Check sheet for the modelled part. Datum: model origin and axes. Units: mm. A direction names the side the tool comes from. Coordinates: 2 decimals unless noted, no trailing zeros. Write each loop counter-clockwise with the first axis right and the second up, starting at its lowest first coordinate (ties: lowest second). Pieces come first, ordered by that corner, then holes. Notation, with made-up numbers: (67, 20.25) -> (105, 20.25) arc R16 ccw to (105, 39.25) -> close; hole circle Ø10 at (84, -1.75). An arc over 180 degrees is marked (long way). One line per item, written item: value. Start each with the question number.
1) Gauge pin test, flat ends, axial feed: P1, Ø5, axis at x = 6, y = -2.5, coming from the +Z side (3 decimals); P2, Ø2.5, axis at y = -2.5, z = -2.5, coming from the +X side. Record the tip position at first contact, or that the pin passes through.
2) Set-up check for faces 1 (the flat face through (12, 0, -8.255)), 2 (the flat face through (2.54, 4.762, -8.44)): record each of +Z, -Z, +X, -X, +Y, -Y from which the full face is reachable in a straight line by a thin tool's end or side.
3) Sectioned sample at B-B on y = 0. Enter the section's corners in (x, z) (1 decimal).
4) Sectioned sample at A-A on x = 15.24. Enter the section's corners in (y, z) (1 decimal), plus the area to 3 significant figures.
5) Sectioned sample at D-D on y = -4. Enter the section's corners in (x, z) (1 decimal), plus the area to 3 significant figures.
6) Draft check along Y on faces 3 (the cylindrical face through (13.09, 0.09, -10.92)), 4 (the flat face through (0, 0, -4)), 5 (the flat face through (2.54, -4.762, -8.44)). Enter one of: +Y half, -Y half, draft (parallel to the pull), parting line (faces both ways), or undercut.
7) Scan lines: line 1 along Y through (x, z) = (15.24, -10.4); line 2 along Z through (x, y) = (2, -1.75) (1 decimal); line 3 along Y through (x, z) = (-6, -4.5). Record each from-to range of solid material in increasing order. Write a range as [from, to].
8) Sectioned sample at C-C on z = -2. Enter the section's corners in (x, y) (1 decimal).
```python
from build123d import *

# Parameters (mm, degrees)
BOSS_EXTRUDE1_DEPTH = 4.7625
SKETCH3_R           = 2.15265
CUT_EXTRUDE1_DEPTH  = 29.13057167


with BuildPart() as part:
    # Sketch1 → Boss-Extrude1 (new, symmetric)
    with BuildSketch(Plane(origin=(0, 0, 0), x_dir=(1, 0, 0), z_dir=(0, 1, 0))):
        Polygon((0, 0), (0, 8.255), (24.13, 8.255), (24.13, 13.6525), (-10.795, 13.6525), (-10.795, 0), align=None)
    extrude(amount=BOSS_EXTRUDE1_DEPTH, both=True)

    # Sketch3 → Cut-Extrude1 (cut, through all)
    with BuildSketch(Plane.XY):
        with Locations((15.24, 0)):
            Circle(SKETCH3_R)
        with Locations((-5.3975, 0)):
            Circle(SKETCH3_R)
    extrude(amount=-CUT_EXTRUDE1_DEPTH, mode=Mode.SUBTRACT)


solid = part.part
```
Answers:
1. P1: stops at z = -8.255
1. P2: stops at x = 0
2. face 1: +Z, +X, +Y, -Y
2. face 2: +Z, -Z, +X, -X, +Y
3. outline: (-10.8, -13.7) -> (-7.6, -13.7) -> (-7.6, 0) -> (-10.8, 0) -> close; (-3.2, -13.7) -> (13.1, -13.7) -> (13.1, -8.3) -> (0, -8.3) -> (0, 0) -> (-3.2, 0) -> close; (17.4, -13.7) -> (24.1, -13.7) -> (24.1, -8.3) -> (17.4, -8.3) -> close
4. outline: (-4.8, -13.7) -> (-2.2, -13.7) -> (-2.2, -8.3) -> (-4.8, -8.3) -> close; (2.2, -13.7) -> (4.8, -13.7) -> (4.8, -8.3) -> (2.2, -8.3) -> close
4. area: 28.2 mm2
5. outline: (-10.8, -13.7) -> (24.1, -13.7) -> (24.1, -8.3) -> (0, -8.3) -> (0, 0) -> (-10.8, 0) -> close
5. area: 278 mm2
6. face 3: undercut
6. face 4: draft
6. face 5: -Y half
7. line 1: y = [-4.76, -2.15], [2.15, 4.76]
7. line 2: z = [-13.7, -8.3]
7. line 3: y = [-4.76, -2.07], [2.07, 4.76]
8. outline: (-10.8, -4.8) -> (0, -4.8) -> (0, 4.8) -> (-10.8, 4.8) -> close; hole circle Ø4.3 at (-5.4, 0)
